The drawing under review shows one solid part. Ordinate dimensions are in mm from its lowest x, y, z. A direction names the side the tool comes from. Give positions to 0.01 mm unless a question says otherwise; leave off trailing zeros. Write each loop counter-clockwise with the first axis right and the second up, starting at its lowest first coordinate (ties: lowest second). Pieces come first, ordered by that corner, then holes. Notation, with made-up numbers: M -11,13 L 3,13 A19 ccw 3,50 Z; hole C 44.25,-23 d2. An arc over 180 degrees is marked long. Write item = value, one per line. Start each with the question number.
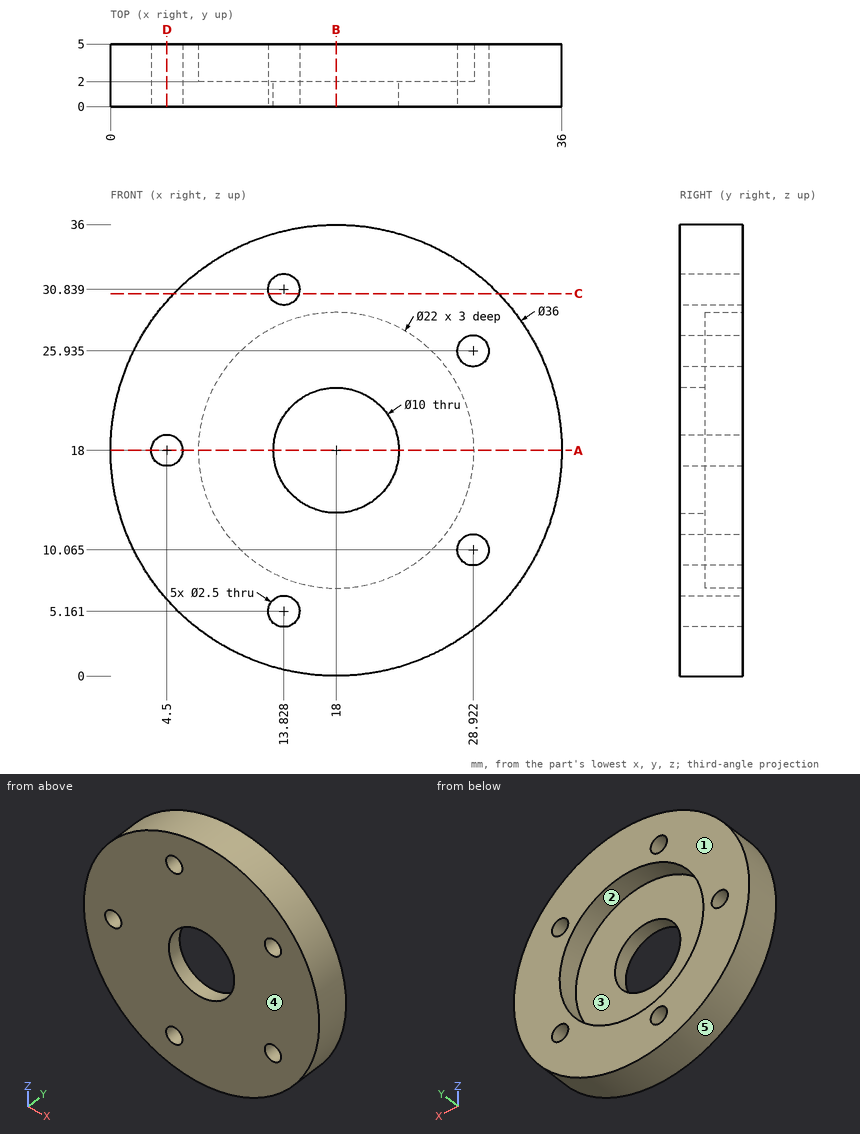
Item 1: To check wall thickness, follow probe 1 along X at (y, z) = (0.7, 18); probe 2 along X at (y, z) = (4.3, 18); probe 3 along X at (y, z) = (3.8, 15). State the ranges of each line that lie inside material, in increasing order. Write a range as [from, to].
Item 2: We need section B-B, the plane x = 18. Write out the cut boundary in (y, z), and give its area (3 significant figures).
Item 3: We need section D-D, the plane x = 4.5. Write out the cut boundary in (y, z), and give its area (3 significant figures).
Item 4: We need section A-A, the plane z = 18. Write out the cut boundary in (x, y).
Item 5: We need section C-C, the plane z = 30.5. Write out the cut boundary in (x, y) (1 decimal).
Item 6: For the marked faces 1 and 2, list the 3-axis set-ups (+Z, -Z, +X, -X, +Y, -Y) from which the entire face can be reached by the end or side of a thin tool; tool diameter is ignored.
Item 7: Clearance check with flat-ended pins moving along their axes: P1, Ø17.5, axis at x = 15, z = 18, coming from the +Y side; P2, Ø2, axis at y = 3.5, z = 13, coming from the +X side; P3, Ø1.5, axis at y = 3.5, z = 17.5, coming from the -X side; P4, Ø1.5, axis at x = 28.92, z = 25.94, coming from the -Y side. State where each tip first meets the part, or that it passes through.
Item 8: The part is to be moulded in two halves that separate along Z. For the marked faces 3, 4 and 5, say which applies: released by +Z, released by -Z, zero draft, split by the parting line, or undercut.
Worked out:
q1.probe_1 = [0, 3.25], [5.75, 13], [23, 36]
q1.probe_2 = [0, 3.25], [5.75, 7], [29, 36]
q1.probe_3 = [0.25, 7.42], [28.58, 35.75]
q2.outline = M 0,0 L 5,0 L 5,7 L 2,7 L 2,13 L 0,13 Z; M 0,23 L 2,23 L 2,29 L 5,29 L 5,36 L 0,36 Z
q2.area = 94.0 mm²
q3.outline = M 0,6.09 L 5,6.09 L 5,16.75 L 0,16.75 Z; M 0,19.25 L 5,19.25 L 5,29.91 L 0,29.91 Z
q3.area = 107 mm²
q4.outline = M 0,0 L 3.25,0 L 3.25,5 L 0,5 Z; M 5.75,0 L 13,0 L 13,2 L 7,2 L 7,5 L 5.75,5 Z; M 23,0 L 36,0 L 36,5 L 29,5 L 29,2 L 23,2 Z
q5.outline = M 5,0 L 12.6,0 L 12.6,5 L 5,5 Z; M 15,0 L 31,0 L 31,5 L 15,5 Z
q6.face_1 = +Z, -Z, +X, -X, +Y
q6.face_2 = +Y
q7.P1 = 5
q7.P2 = 35.55
q7.P3 = 0
q7.P4 = through
q8.face_3 = undercut
q8.face_4 = zero draft
q8.face_5 = split by the parting line
